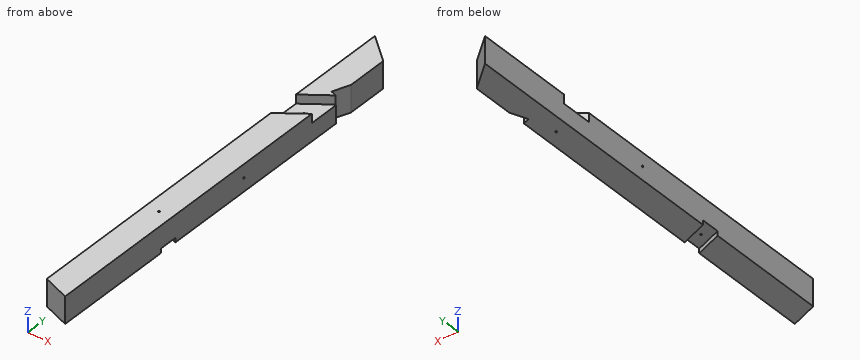
from build123d import *

# Parameters (mm, degrees)
SKETCH1_W           = 150
SKETCH1_H           = 150
BOSS_EXTRUDE1_DEPTH = 1250
SKETCH2_R           = 5
CUT_EXTRUDE1_DEPTH  = 1262.199825563
ROOFCUT_DEPTH       = 1262.199825563
TOPCUT_DEPTH        = 1262.199825563
SKETCH5_R           = 5
CUT_EXTRUDE4_DEPTH  = 1262.199825563
CUT_EXTRUDE5_DEPTH  = 50
CUT_EXTRUDE6_DEPTH  = 25
CUT_EXTRUDE7_DEPTH  = 1262.199825563


with BuildPart() as part:
    # Sketch1 → Boss-Extrude1 (new, symmetric)
    with BuildSketch(Plane(origin=(0, 0, 0), x_dir=(1, 0, 0), z_dir=(0, 1, 0))):
        Rectangle(SKETCH1_W, SKETCH1_H)
    extrude(amount=BOSS_EXTRUDE1_DEPTH, both=True)

    # Sketch2 → Cut-Extrude1 (cut, through all)
    with BuildSketch(Plane.XY.offset(75)):
        with Locations((0, 610)):
            Circle(SKETCH2_R)
        with Locations((0, -460)):
            Circle(SKETCH2_R)
    extrude(amount=-CUT_EXTRUDE1_DEPTH, mode=Mode.SUBTRACT)

    # Sketch3 → RoofCut (cut, through all)
    with BuildSketch(Plane.XY.offset(75)):
        Polygon((-75, 1232.703797136), (75, 1097.593747534), (75, 1250), (-75, 1250), align=None)
    extrude(amount=-ROOFCUT_DEPTH, mode=Mode.SUBTRACT)

    # Sketch4 → TopCut (cut, through all)
    with BuildSketch(Plane.XY.offset(75)):
        Polygon((75, 858.878428235), (37.522465852, 764.870707964), (75, 749.720866047), align=None)
    extrude(amount=-TOPCUT_DEPTH, mode=Mode.SUBTRACT)

    # Sketch5 → Cut-Extrude4 (cut, through all)
    with BuildSketch(Plane(origin=(75, 0, 0), x_dir=(0, 0, -1), z_dir=(1, 0, 0))):
        with Locations((0, 70)):
            Circle(SKETCH5_R)
    extrude(amount=-CUT_EXTRUDE4_DEPTH, mode=Mode.SUBTRACT)

    # Sketch7 → Cut-Extrude5 (cut)
    with BuildSketch(Plane.XY.offset(75)):
        Polygon((-75, 649.486666068), (-75, 465.302341615), (75, 571.125839473), (75, 754.950569225), align=None)
    extrude(amount=-CUT_EXTRUDE5_DEPTH, mode=Mode.SUBTRACT)

    # Sketch8 → Cut-Extrude6 (cut)
    with BuildSketch(Plane(origin=(0, 0, -75), x_dir=(-1, 0, 0), z_dir=(0, 0, -1))):
        Polygon((-78.608377022, -545.707193758), (75, -483.612856927), (75, -375.751449205), (-75, -436.387143073), align=None)
    extrude(amount=-CUT_EXTRUDE6_DEPTH, mode=Mode.SUBTRACT)

    # Sketch9 → Cut-Extrude7 (cut, through all)
    with BuildSketch(Plane.XY.offset(75)):
        Polygon((-75, -1189.364306132), (75, -1250), (-75, -1250), align=None)
    extrude(amount=-CUT_EXTRUDE7_DEPTH, mode=Mode.SUBTRACT)


solid = part.part
Geometry: final body of the model. Coordinates: model frame, mm. Round coordinates to 2 decimals unless told otherwise and drop trailing zeros. Order: outer loops, then holes, each group sorted by start corner. A loop starts at its lowest first (then second) coordinate and runs counter-clockwise, first axis right, second up.
Q1. Pin query (flat end, axial travel): pin 1 (3 mm diameter, centred on x = -22.5, z = 35.5, fed in from -Y); pin 2 (8 mm diameter, centred on x = 0, y = 610, fed in from +Z); pin 3 (13 mm diameter, centred on x = 0, y = -460, fed in from -Z); pin 4 (1 mm diameter, centred on x = -29.5, z = 5.5, fed in from -Y). Return the tip coordinate at first contact, or that it passes through.
Result sheet:
pin 1: stops at y = -1211.19
pin 2: passes through
pin 3: stops at z = -50
pin 4: stops at y = -1207.96
Q2. Material intervals for probe 1 along Y at (x, z) = (0, 48.5); probe 2 along X at (y, z) = (610, -41); probe 3 along Z at (x, y) = (-8.5, 606.5), sorted ascending.
Result sheet:
probe 1: y = -1219.68 to -465, -455 to 518.21, 702.22 to 1165.15
probe 2: x = -75 to -5, 5 to 75
probe 3: z = -75 to 25
Q3. Section A-A, the plane y = 793.5. Output: boundary loops of the cut face in (x, z).
Result sheet:
outline: (-75, -75) - (48.94, -75) - (48.94, 75) - (-75, 75) - close
